Source: CAD feature listing. Evaluate the final solid. Frame: model axes, mm. A direction names the side the tool comes from. Give positions to 0.01 mm unless a question says otherwise; leave off trailing zeros. Order: outer loops, then holes, each group sorted by start corner. A loop starts at its lowest first (then second) coordinate and runs counter-clockwise, first axis right, second up. Notation, with made-up numbers: M -40,-6 L 18,-6 A20 cw 18,4 Z; hole C -19.5,8 d2. An arc over 180 degrees is marked long. Answer as a JSON object with one key per item and string values. Group by question number.
1. Pull-direction query (Z, two-part tool) for faces 4 (the flat face through (0, 609.557, -1)), 5 (the flat face through (-7.5, 344, -1)), 6 (the flat face through (0, 344, 75)); classes: +Z half, -Z half, draft (parallel to the pull), parting line (faces both ways), or undercut.
2. Pin query (flat end, axial travel): P1, Ø8, axis at y = 192.5, z = -18, coming from the -X side; P2, Ø24, axis at y = 122.73, z = 0, coming from the -X side. Return the tip coordinate at first contact, or that it passes through.
3. Section query B-B (x = -13). Output: boundary loops of the cut face in (y, z), plus the area to 3 significant figures.
4. Section query D-D (z = -28). Output: boundary loops of the cut face in (x, y), plus the area to 3 significant figures.
5. Material intervals for L1, parallel to Y at x = 4.25, z = 0; L2, parallel to Z at x = -15, y = 403; L3, parallel to Y at x = 1, z = -5, sorted ascending. Write a range as [from, to].
6. Section query C-C (y = 402). Output: boundary loops of the cut face in (x, z), plus the area to 3 significant figures.
7. Set-up query: faces 1 (the flat face through (7.5, 344, 1)), 2 (the flat face through (-13, 344, 56.25)), 3 (the flat face through (18.75, 344, -65)). Return all of +Z, -Z, +X, -X, +Y, -Y with unobstructed straight access to the full face (end or side cutting, diameter ignored); none if empty.
8. Section query A-A (z = 0). Output: boundary loops of the cut face in (x, y).
from build123d import *

# Parameters (mm, degrees)
BOSS_EXTRUDE1_DEPTH = 699.106666667
SKETCH2_R           = 50
SKETCH2_R_2         = 20
CUT_EXTRUDE1_DEPTH  = 1000
SCALE1_SCALE        = 0.75


with BuildPart() as part:
    # Sketch1 → Boss-Extrude1 (new body)
    with BuildSketch(Plane(origin=(0, 0, 0), x_dir=(1, 0, 0), z_dir=(0, 1, 0))):
        Polygon((-25, -75), (-25, -100), (25, -100), (25, -75), (10, -75), (10, 75), (25, 75), (25, 100), (-25, 100), (-25, 75), (-10, 75), (-10, -75), align=None)
    extrude(amount=BOSS_EXTRUDE1_DEPTH)

    # Sketch2 → Cut-Extrude1 (cut)
    with BuildSketch(Plane(origin=(10, 0, 0), x_dir=(0, 0, -1), z_dir=(1, 0, 0))):
        with Locations((0, 599.106666667)):
            Circle(SKETCH2_R)
        with Locations((0, 50)):
            Circle(SKETCH2_R_2)
    extrude(amount=-CUT_EXTRUDE1_DEPTH, mode=Mode.SUBTRACT)


with BuildPart() as part_1:
    # Scale1: scaled about (0, 340.906804135, 0)
    add(part.part.scale(SCALE1_SCALE).moved(Location((0, 85.226701034, 0))))


solid = part_1.part
Answer sheet:
{
 "1": {"face 4": "draft", "face 5": "undercut", "face 6": "+Z half"},
 "2": {"P1": "x = -7.5", "P2": "through"},
 "3": {"outline": "M 85.23,-75 L 609.56,-75 L 609.56,-56.25 L 85.23,-56.25 Z; M 85.23,56.25 L 609.56,56.25 L 609.56,75 L 85.23,75 Z", "area": "19,700 mm^2"},
 "4": {"outline": "M -7.5,85.23 L 7.5,85.23 L 7.5,509.61 L -7.5,509.61 Z; M -7.5,559.5 L 7.5,559.5 L 7.5,609.56 L -7.5,609.56 Z", "area": "7,120 mm^2"},
 "5": {"L1": "[85.23, 107.73], [137.73, 497.06], [572.06, 609.56]", "L2": "[-75, -56.25], [56.25, 75]", "L3": "[85.23, 108.58], [136.87, 497.39], [571.72, 609.56]"},
 "6": {"outline": "M -18.75,-75 L 18.75,-75 L 18.75,-56.25 L 7.5,-56.25 L 7.5,56.25 L 18.75,56.25 L 18.75,75 L -18.75,75 L -18.75,56.25 L -7.5,56.25 L -7.5,-56.25 L -18.75,-56.25 Z", "area": "3,090 mm^2"},
 "7": {"face 1": "+X, +Y, -Y", "face 2": "-X, +Y, -Y", "face 3": "+Z, -Z, +X, +Y, -Y"},
 "8": {"outline": "M -7.5,85.23 L 7.5,85.23 L 7.5,107.73 L -7.5,107.73 Z; M -7.5,137.73 L 7.5,137.73 L 7.5,497.06 L -7.5,497.06 Z; M -7.5,572.06 L 7.5,572.06 L 7.5,609.56 L -7.5,609.56 Z"}
}
